Here's how the part is built. I have some questions about the finished solid (model axes, mm). A direction names the side the tool comes from. Give positions to 0.01 mm unless a question says otherwise; leave off trailing zeros. Write each loop counter-clockwise with the first axis right and the second up, starting at its lowest first coordinate (ties: lowest second). Pieces come first, ordered by that corner, then holes. Notation, with made-up numbers: (61.5, 13) - (83.5, 13) arc R31 ccw to (83.5, 42) - close; hole circle Ø4 at (78.25, -21). An arc over 180 degrees is marked (long way). One line per item, written item: value. Start each with the question number.
1) Please list where these lines run through material, in increasing order: L1, parallel to X at y = 1.25, z = -44.18; L2, parallel to Z at x = 24, y = 17.25; L3, parallel to X at y = 15.25, z = -41. Write a range as [from, to].
2) Imagine slicing it at B-B on z = -44.18. Write out the boundary of the cut face in (x, y), plus the area to 3 significant figures.
3) We'd pull the mould along X, two halves only. Please class faces 1 (the flat face through (0, 10, -44)), 2 (the flat face through (68, 11.1, -61.6)), 3 (the flat face through (26, 10, -87)): +X half, -X half, draft (parallel to the pull), parting line (faces both ways), or undercut.
4) On a 3-axis mill with a long thin cutter (end or side, diameter ignored), from which of +Z, -Z, +X, -X, +Y, -Y can I reach the whole of each face in a straight line? I mean faces 4 (the flat face through (52, 10, -82)), 5 (the flat face through (58, 11, -61)), 6 (the flat face through (49, 20, -44)), 7 (the flat face through (70, 11, -61.85)), 8 (the flat face through (62, 10, -57)). Say none if no direction works.
5) Imagine slicing it at D-D on y = 5. Write out the boundary of the cut face in (x, z), plus the area to 3 significant figures.
6) I'm going to push flat-ended pins straight in: P1, Ø8, axis at x = 61.5, y = 15, coming from the -Z side; P2, Ø0.7, axis at x = 49.5, z = -75, coming from the +Y side; P3, Ø10, axis at x = 35, z = -38, coming from the +Y side. Where does each tip first touch, or does it pass through?
7) Imagine slicing it at A-A on x = 21.56. Write out the boundary of the cut face in (y, z), plus the area to 3 significant figures.
8) Imagine slicing it at C-C on y = 14.5. Count the separate pieces of the cut face and the enclosed holes in it, plus the area to 3 significant figures.
from build123d import *

# Parameters (mm, degrees)
BOSS_EXTRUDE1_DEPTH = 20
SKETCH2_W           = 44
SKETCH2_H           = 79
BATTERY_CUT_DEPTH   = 18
SKETCH3_W           = 20
SKETCH3_H           = 12
CUT_EXTRUDE2_DEPTH  = 18
SKETCH4_R           = 1.1
NUT_HOLES_DEPTH     = 10
SKETCH5_W           = 10.3
SKETCH5_H           = 15
CUT_EXTRUDE4_DEPTH  = 5
SKETCH6_R           = 1.6
CUT_EXTRUDE5_DEPTH  = 6
FILLET1_R           = 2


with BuildPart() as part:
    # Sketch1 → Boss-Extrude1 (new body)
    with BuildSketch(Plane(origin=(0, 0, 0), x_dir=(1, 0, 0), z_dir=(0, 1, 0))):
        Polygon((52, 77), (52, 87), (0, 87), (0, 0), (52, 0), (52, 57), (72, 57), (72, 77), align=None)
    extrude(amount=BOSS_EXTRUDE1_DEPTH)

    # Sketch2 → battery cut (cut)
    with BuildSketch(Plane(origin=(0, 20, 0), x_dir=(1, 0, 0), z_dir=(0, 1, 0))):
        with Locations((26, 43.5)):
            Rectangle(SKETCH2_W, SKETCH2_H)
    extrude(amount=-BATTERY_CUT_DEPTH, mode=Mode.SUBTRACT)

    # Sketch3 → Cut-Extrude2 (cut)
    with BuildSketch(Plane(origin=(0, 20, 0), x_dir=(1, 0, 0), z_dir=(0, 1, 0))):
        with Locations((58, 67)):
            Rectangle(SKETCH3_W, SKETCH3_H)
    extrude(amount=-CUT_EXTRUDE2_DEPTH, mode=Mode.SUBTRACT)

    # Sketch4 → nut holes (cut)
    with BuildSketch(Plane(origin=(0, 20, 0), x_dir=(1, 0, 0), z_dir=(0, 1, 0))):
        with Locations((4, 2)):
            Circle(SKETCH4_R)
        with Locations((48, 2)):
            Circle(SKETCH4_R)
        with Locations((24, 85)):
            Circle(SKETCH4_R)
        with Locations((50, 75)):
            Circle(SKETCH4_R)
    extrude(amount=-NUT_HOLES_DEPTH, mode=Mode.SUBTRACT)

    # Sketch5 → Cut-Extrude4 (cut)
    with BuildSketch(Plane(origin=(72, 0, 0), x_dir=(0, 0, -1), z_dir=(1, 0, 0))):
        with Locations((67, 11.5)):
            Rectangle(SKETCH5_W, SKETCH5_H)
    extrude(amount=-CUT_EXTRUDE4_DEPTH, mode=Mode.SUBTRACT)

    # Sketch6 → Cut-Extrude5 (cut)
    with BuildSketch(Plane(origin=(0, 2, 0), x_dir=(1, 0, 0), z_dir=(0, 1, 0))):
        with Locations((21.56, 44.18)):
            Circle(SKETCH6_R)
        with Locations((43.53, 44.18)):
            Circle(SKETCH6_R)
        with Locations((38, 44.18)):
            Circle(SKETCH6_R)
        with Locations((16.03, 44.18)):
            Circle(SKETCH6_R)
    extrude(amount=-CUT_EXTRUDE5_DEPTH, mode=Mode.SUBTRACT)

    # Fillet1
    fillet1_edges = [part.edges().sort_by_distance(p)[0] for p in [
        (0, 10, -87),
        (52, 10, -87),
        (52, 10, -77),
        (72, 10, -77),
        (72, 10, -57),
        (52, 10, -57),
        (52, 10, 0),
        (0, 10, 0),
    ]]
    fillet(fillet1_edges, radius=FILLET1_R)


solid = part.part
Numbers:
1. L1: [0, 14.43], [17.63, 19.96], [23.16, 36.4], [39.6, 41.93], [45.13, 52]
1. L2: [-87, -86.1], [-83.9, -83], [-4, 0]
1. L3: [0, 4], [48, 52]
2. outline: (0, 0) - (14.43, 0) - (14.43, 2) - (4, 2) - (4, 20) - (0, 20) - close; (17.63, 0) - (19.96, 0) - (19.96, 2) - (17.63, 2) - close; (23.16, 0) - (36.4, 0) - (36.4, 2) - (23.16, 2) - close; (39.6, 0) - (41.93, 0) - (41.93, 2) - (39.6, 2) - close; (45.13, 0) - (52, 0) - (52, 20) - (48, 20) - (48, 2) - (45.13, 2) - close
2. area: 222 mm^2
3. face 1: -X half
3. face 2: undercut
3. face 3: draft
4. face 4: -Z, +X, +Y, -Y
4. face 5: +Y
4. face 6: +Z, -Z, +X, -X, +Y
4. face 7: +X
4. face 8: +Z, +X, +Y, -Y
5. outline: (0, -85) arc R2 ccw to (2, -87) - (50, -87) arc R2 ccw to (52, -85) - (52, -79) arc R2 cw to (54, -77) - (70, -77) arc R2 ccw to (72, -75) - (72, -72.15) - (68, -72.15) - (68, -73) - (48, -73) - (48, -83) - (4, -83) - (4, -4) - (48, -4) - (48, -61) - (68, -61) - (68, -61.85) - (72, -61.85) - (72, -59) arc R2 ccw to (70, -57) - (54, -57) arc R2 cw to (52, -55) - (52, -2) arc R2 ccw to (50, 0) - (2, 0) arc R2 ccw to (0, -2) - close
5. area: 1,160 mm^2
6. P1: z = -77
6. P2: y = 10
6. P3: y = 2
7. outline: (0, -87) - (20, -87) - (20, -83) - (2, -83) - (2, -45.78) - (0, -45.78) - close; (0, -42.58) - (2, -42.58) - (2, -4) - (20, -4) - (20, 0) - (0, 0) - close
7. area: 312 mm^2
8. separate pieces: 1
8. enclosed holes: 4
8. area: 1,150 mm^2
